Geometry: final body of the model. Coordinates: model frame, mm. A direction names the side the tool comes from. Coordinates: 2 decimals unless noted, no trailing zeros. Loops run counter-clockwise (first coordinate to the right, second up) from the corner with the lowest first, then second, coordinate; pieces in that order, holes last. Notation, with made-up numbers: M 42,9.5 L 92,9.5 A33 cw 92,44.5 Z; hole C 57,61 d4. An arc over 180 degrees is marked long. Write each question's results on one line, items separated by ' | '. Start each with the question number.
from build123d import *

# Parameters (mm, degrees)
SKETCH1_W           = 35
SKETCH1_H           = 76.2
BOSS_EXTRUDE1_DEPTH = 3
SKETCH2_W           = 3
SKETCH2_H           = 15
CUT_EXTRUDE1_DEPTH  = 73.446802019
LPATTERN1_COUNT     = 3
LPATTERN1_PITCH     = 22.8
SKETCH3_W           = 3
SKETCH3_H           = 15
CUT_EXTRUDE2_DEPTH  = 73.446802019
LPATTERN2_COUNT     = 3
LPATTERN2_PITCH     = 22.8


with BuildPart() as part:
    # Sketch1 → Boss-Extrude1 (new body)
    with BuildSketch(Plane.XY):
        with Locations((-23.493460648, -21.557986111)):
            Rectangle(SKETCH1_W, SKETCH1_H)
    extrude(amount=BOSS_EXTRUDE1_DEPTH)

    # Sketch2 → Cut-Extrude1 (cut, through all)
    with BuildSketch(Plane.XY.offset(3)):
        with Locations((-39.493460648, 1.242013889)):
            Rectangle(SKETCH2_W, SKETCH2_H)
        with Locations((-7.493460648, 1.242013889)):
            Rectangle(SKETCH2_W, SKETCH2_H)
    cut_extrude1 = extrude(amount=-CUT_EXTRUDE1_DEPTH, mode=Mode.SUBTRACT)

    # LPattern1: Cut-Extrude1 ×3
    with Locations(*[(0, -i * LPATTERN1_PITCH, 0) for i in range(1, LPATTERN1_COUNT)]):
        add(cut_extrude1, mode=Mode.SUBTRACT)

    # Sketch3 → Cut-Extrude2 (cut, through all)
    with BuildSketch(Plane.XY.offset(3)):
        with Locations((-15.493460648, 1.242013889)):
            Rectangle(SKETCH3_W, SKETCH3_H)
    cut_extrude2 = extrude(amount=-CUT_EXTRUDE2_DEPTH, mode=Mode.SUBTRACT)

    # LPattern2: Cut-Extrude2 ×3
    with Locations(*[(0, -i * LPATTERN2_PITCH, 0) for i in range(1, LPATTERN2_COUNT)]):
        add(cut_extrude2, mode=Mode.SUBTRACT)


solid = part.part
Item 1: Section A-A, the plane y = -15. Return loops of the section in (x, z), plus the area to 3 significant figures.
Item 2: Ray query, L1, parallel to X at y = -15, z = 2.8; L2, parallel to Y at x = -38.5, z = 1.1. Return the intervals inside material, ascending. Write a range as [from, to].
Item 3: Contact query for flat-ended pins moving along their axis: P1, Ø1.5, axis at y = 0.5, z = 2, coming from the -X side; P2, Ø0.9, axis at y = -41, z = 1.5, coming from the +X side. Output: stop coordinate, or through.
Item 4: Section B-B, the plane z = 1.7. Count the separate pieces of the cut face and the enclosed holes in it, plus the area to 3 significant figures.
Item 5: Pull-direction query (Y, two-part tool) for faces 4 (the flat face through (-24, -59.658, 1)), 5 (the flat face through (-5.993, -33, 1)), 6 (the flat face through (-40, -36.858, 2)); classes: released by +Y, released by -Y, zero draft, split by the parting line, or undercut.
Item 6: Set-up query: faces 1 (the flat face through (-8.993, -22, 2)), 2 (the flat face through (-16, -14.058, 2)), 3 (the flat face through (-37.993, -44, 2)). Return all of +Z, -Z, +X, -X, +Y, -Y with unobstructed straight access to the full face (end or side cutting, diameter ignored); none if empty.
Solutions:
1) outline: M -37.99,0 L -16.99,0 L -16.99,3 L -37.99,3 Z; M -13.99,0 L -8.99,0 L -8.99,3 L -13.99,3 Z | area: 78.0 mm²
2) L1: x = [-37.99, -16.99], [-13.99, -8.99] | L2: y = [-59.66, -51.86], [-36.86, -29.06], [-14.06, -6.26], [8.74, 16.54]
3) P1: stops at x = -37.99 | P2: stops at x = -8.99
4) separate pieces: 1 | enclosed holes: 3 | area: 2,260 mm²
5) face 4: released by -Y | face 5: zero draft | face 6: undercut
6) face 1: +Z, -Z, +X | face 2: +Z, -Z | face 3: +Z, -Z, -X
